The listing builds one solid part. Answer for the finished solid, in the listing's coordinates (mm). A direction names the side the tool comes from. Give positions to 0.01 mm unless a question says otherwise; leave off trailing zeros. Loops run counter-clockwise (first coordinate to the right, second up) from the corner with the lowest first, then second, coordinate; pieces in that order, holes last. Notation, with made-up numbers: (23, -8.75) - (80, -8.75) arc R15 ccw to (80, 1.25) - close; hole circle Ø3 at (-12, 47). An arc over 180 degrees is marked (long way). One line per item, written item: value. Start each with the question number.
from build123d import *

# Parameters (mm, degrees)
POT_BASE_SKETCH_R   = 130
POT_BASE_DEPTH      = 15
POT_WALL_SKETCH_R   = 130
POT_WALL_SKETCH_R_2 = 115
POT_WALL_DEPTH      = 250
POT_START           = 238
POT_RIM_SKETCH_R    = 150
POT_RIM_SKETCH_R_2  = 115
POT_RIM_DEPTH       = 12


with BuildPart() as part:
    # Pot Base Sketch → Pot Base (new body)
    with BuildSketch(Plane(origin=(0, 0, 0), x_dir=(1, 0, 0), z_dir=(0, 1, 0))):
        with Locations(Location((0, 0, 0), (0, 0, 270))):
            Circle(POT_BASE_SKETCH_R)
    extrude(amount=POT_BASE_DEPTH)

    # Pot Wall Sketch → Pot Wall (add)
    with BuildSketch(Plane(origin=(0, 0, 0), x_dir=(1, 0, 0), z_dir=(0, 1, 0))):
        with Locations(Location((0, 0, 0), (0, 0, 270))):
            Circle(POT_WALL_SKETCH_R)
        with Locations(Location((0, 0, 0), (0, 0, 270))):
            Circle(POT_WALL_SKETCH_R_2, mode=Mode.SUBTRACT)
    extrude(amount=POT_WALL_DEPTH)

    # Pot Rim Sketch → Pot Rim (add)
    with BuildSketch(Plane(origin=(0, 0, 0), x_dir=(1, 0, 0), z_dir=(0, 1, 0)).offset(POT_START)):
        with Locations(Location((0, 0, 0), (0, 0, 270))):
            Circle(POT_RIM_SKETCH_R)
        with Locations(Location((0, 0, 0), (0, 0, 270))):
            Circle(POT_RIM_SKETCH_R_2, mode=Mode.SUBTRACT)
    extrude(amount=POT_RIM_DEPTH)


solid = part.part
1. A cutting plane is placed at B-B (y = 96.5). Determine the outline of the cut face in (x, z).
2. Determine the mould class of faces 1 (the flat face through (2, 0, -2)), 2 (the cylindrical face through (-112.265, 130.855, -24.93)), 3 (the cylindrical face through (-91.273, 243.916, -119.035)) for opening direction X: released by +X, released by -X, zero draft, split by the parting line, or undercut.
3. A cutting plane is placed at C-C (x = 62.5). Determine the outline of the cut face in (y, z).
4. Find the intervals of material crossed by L1, parallel to Z at x = 0, y = 189; L2, parallel to Y at x = 35.5, z = -18.5, in increasing order. Write a range as [from, to].
5. A cutting plane is placed at A-A (z = 0). Determine the outline of the cut face in (x, y).
6. For faces 4 (the flat face through (2, 15, -2)), 5 (the flat face through (123, 238, -45)), 6 (the flat face through (-110.4, 250, -34)), determine the directions among +Z, -Z, +X, -X, +Y, -Y from which every point of the face is accessible in a straight line to the end or side of a thin tool.
7. Flat-ended cylindrical pins translate along their axes: pin 1 (8 mm diameter, centred on x = -27, y = 153, fed in from +Z); pin 2 (8 mm diameter, centred on x = 6, y = 120.5, fed in from +Z); pin 3 (8 mm diameter, centred on x = 57.5, z = 52.5, fed in from +Y); pin 4 (8 mm diameter, centred on x = 75.5, z = -56, fed in from -Y). Find the tip coordinate at first contact, or state that the pin passes through.
Results below:
1. outline: circle Ø260 at (0, 0); hole circle Ø230 at (0, 0)
2. face 1: zero draft
2. face 2: undercut
2. face 3: split by the parting line
3. outline: (0, -113.99) - (238, -113.99) - (238, -136.36) - (250, -136.36) - (250, -96.53) - (15, -96.53) - (15, 96.53) - (250, 96.53) - (250, 136.36) - (238, 136.36) - (238, 113.99) - (0, 113.99) - close
4. L1: z = [-130, -115], [115, 130]
4. L2: y = [0, 15]
5. outline: (-150, 238) - (-130, 238) - (-130, 0) - (130, 0) - (130, 238) - (150, 238) - (150, 250) - (115, 250) - (115, 15) - (-115, 15) - (-115, 250) - (-150, 250) - close
6. face 4: +Y
6. face 5: -Y
6. face 6: +Z, -Z, +X, -X, +Y
7. pin 1: stops at z = 127.95
7. pin 2: stops at z = 129.98
7. pin 3: stops at y = 15
7. pin 4: stops at y = 0
